Input: part model. Units: mm. Frame: model coordinates. A direction names the side the tool comes from. Coordinates: 2 decimals unless noted, no trailing zeros. Loops run counter-clockwise (first coordinate to the right, second up) from the corner with the lowest first, then second, coordinate; pieces in that order, holes last. Notation, with made-up numbers: (64, 44.5) -> (102, 44.5) arc R29 cw to (102, 80.5) -> close; hole circle Ø9 at (87, -38.5). An arc over 180 degrees is marked (long way). Put each result on its own line as item: value. Start each with the question number.
1) Cut plane A-A (y = 9). Return the cut outline in (x, z).
2) Contact query for a flat-ended pin moving along its axis: P1, Ø3, axis at x = -105.9, y = 5.26, coming from the -Z side. Output: stop coordinate, or through.
3) Cut plane D-D (z = 4). State how many separate pieces and enclosed holes the cut face has, plus the area to 3 significant figures.
4) Pull-direction query (X, two-part tool) for faces 3 (the cylindrical face through (62.75, -23.27, 2.71)), 4 (the flat face through (-10, 29.257, 3)), 5 (the flat face through (-14, -29.243, 3)), 6 (the flat face through (-112.397, -7, 3)); classes: pulls with the +X half, pulls with the -X half, needs draft (parallel to the pull), parting line crosses it, or undercut.
5) Cut plane B-B (x = 10). Return the cut outline in (y, z).
6) Cut plane C-C (y = -17.5). Return the cut outline in (x, z).
7) Material intervals for L1, parallel to Y at x = 8.5, z = 3; L2, parallel to X at y = 8.5, z = 1.3; L3, parallel to X at y = -28.5, z = 2.35, sorted ascending.
8) Set-up query: faces 1 (the flat face through (-106, -10.743, 3)), 2 (the flat face through (-10, -30, 5.5)). Return all of +Z, -Z, +X, -X, +Y, -Y with unobstructed straight access to the full face (end or side cutting, diameter ignored); none if empty.
from build123d import *

# Parameters (mm, degrees)
F0_W     = 208
F0_H     = 72
F0_R     = 1.75
F0_W_2   = 6
F0_H_2   = 9
F0_W_3   = 100.394129
F0_H_3   = 42
F0_R_2   = 2
F0_R_3   = 3.75
F1_DEPTH = 5.5


with BuildPart() as f1:
    # F0 (on Top) → F1 (new body)
    with BuildSketch(Plane.XY):
        with Locations((-8.396824, -6.742854)):
            Rectangle(F0_W, F0_H)
        with Locations((-72.564889, -27.742854)):
            Circle(F0_R, mode=Mode.SUBTRACT)
        with Locations((-105.896824, -15.242854)):
            Rectangle(F0_W_2, F0_H_2, mode=Mode.SUBTRACT)
        with Locations((-12.867824, -8.242854)):
            Rectangle(F0_W_3, F0_H_3, mode=Mode.SUBTRACT)
        with Locations((71.82924, -27.742854)):
            Circle(F0_R, mode=Mode.SUBTRACT)
        with Locations((61.82924, -21.492854)):
            Circle(F0_R_2, mode=Mode.SUBTRACT)
        with Locations((89.103176, -15.242854)):
            Rectangle(F0_W_2, F0_H_2, mode=Mode.SUBTRACT)
        with Locations((-105.896824, 5.257146)):
            Circle(F0_R, mode=Mode.SUBTRACT)
        with Locations((-72.564889, 21.757146)):
            Circle(F0_R, mode=Mode.SUBTRACT)
        with Locations((62.07924, -5.242854)):
            Circle(F0_R_3, mode=Mode.SUBTRACT)
        with Locations((89.103176, 4.757146)):
            Circle(F0_R, mode=Mode.SUBTRACT)
        with Locations((71.82924, 21.757146)):
            Circle(F0_R, mode=Mode.SUBTRACT)
    extrude(amount=F1_DEPTH)


solid = f1.part
Results found:
1. outline: (-112.4, 0) -> (-63.06, 0) -> (-63.06, 5.5) -> (-112.4, 5.5) -> close; (37.33, 0) -> (95.6, 0) -> (95.6, 5.5) -> (37.33, 5.5) -> close
2. P1: passes through
3. separate pieces: 1
3. enclosed holes: 11
3. area: 10,500 mm2
4. face 3: undercut
4. face 4: needs draft
4. face 5: undercut
4. face 6: pulls with the -X half
5. outline: (-42.74, 0) -> (-29.24, 0) -> (-29.24, 5.5) -> (-42.74, 5.5) -> close; (12.76, 0) -> (29.26, 0) -> (29.26, 5.5) -> (12.76, 5.5) -> close
6. outline: (-112.4, 0) -> (-108.9, 0) -> (-108.9, 5.5) -> (-112.4, 5.5) -> close; (-102.9, 0) -> (-63.06, 0) -> (-63.06, 5.5) -> (-102.9, 5.5) -> close; (37.33, 0) -> (86.1, 0) -> (86.1, 5.5) -> (37.33, 5.5) -> close; (92.1, 0) -> (95.6, 0) -> (95.6, 5.5) -> (92.1, 5.5) -> close
7. L1: y = -42.74 to -29.24, 12.76 to 29.26
7. L2: x = -112.4 to -63.06, 37.33 to 95.6
7. L3: x = -112.4 to -74.14, -70.99 to -63.06, 37.33 to 70.25, 73.41 to 95.6
8. face 1: +Z, -Z
8. face 2: +Z, +X, -X, +Y, -Y
